Geometry check sheet. Reference: the model listing, model coordinates, mm. Round coordinates to 2 decimals unless told otherwise and drop trailing zeros. Write each loop counter-clockwise with the first axis right and the second up, starting at its lowest first coordinate (ties: lowest second). Pieces come first, ordered by that corner, then holes. Notation, with made-up numbers: (-31.5, -4.75) -> (11.5, -4.75) arc R27 cw to (11.5, 15.25) -> close; hole circle Ø6 at (-10, -8.75). An arc over 180 degrees is marked (long way). One line per question, with ' | ' between items.
Autodesk Inventor part; units mm, degrees
ref_plane "YZ Plane" through (0, 0, 0) normal (1, 0, 0) x (0, 1, 0)
ref_plane "XZ Plane" through (0, 0, 0) normal (0, 1, 0) x (-1, 0, 0)
ref_plane "XY Plane" through (0, 0, 0) normal (0, 0, 1) x (1, 0, 0)
sketch "Sketch1" plane through (0, 0, 0) normal (0, 0, 1) x (1, 0, 0)
  arc A0 (235.6827, -57.867) -> (240.6827, -52.867) centre (235.6827, -52.867) ccw
  line L0 (240.6827, -52.867) -> (240.6827, 24.133)
  arc A1 (240.6827, 24.133) -> (235.6827, 29.133) centre (235.6827, 24.133) ccw
  line L1 (235.6827, 29.133) -> (-24.3173, 29.133)
  arc A2 (-24.3173, 29.133) -> (-29.3173, 24.133) centre (-24.3173, 24.133) ccw
  line L2 (-29.3173, 24.133) -> (-29.3173, -52.867)
  arc A3 (-29.3173, -52.867) -> (-24.3173, -57.867) centre (-24.3173, -52.867) ccw
  line L3 (-24.3173, -57.867) -> (235.6827, -57.867)
  circle A4 centre (235.6827, 23.633) radius 1.7
  circle A5 centre (235.6827, -5.867) radius 1.7
  circle A6 centre (-24.3173, -5.867) radius 1.7
  circle A7 centre (-24.3173, 23.633) radius 1.7
  circle A8 centre (208.6827, 8.133) radius 2.75
  circle A9 centre (228.1827, -46.867) radius 3.3
  circle A10 centre (189.1827, -46.867) radius 3.3
  circle A11 centre (22.1827, -46.867) radius 3.3
  circle A12 centre (-16.8173, -46.867) radius 3.3
  circle A13 centre (235.6827, -5.867) radius 1.7
  circle A14 centre (235.6827, 23.633) radius 1.7
  circle A15 centre (-24.3173, 23.633) radius 1.7
  circle A16 centre (-24.3173, -5.867) radius 1.7
  arc A17 (235.6827, -57.867) -> (240.6827, -52.867) centre (235.6827, -52.867) ccw
  line L4 (240.6827, -52.867) -> (240.6827, 24.133)
  arc A18 (240.6827, 24.133) -> (235.6827, 29.133) centre (235.6827, 24.133) ccw
  line L5 (235.6827, 29.133) -> (172.1827, 29.133)
  arc A19 (-24.3173, 29.133) -> (-29.3173, 24.133) centre (-24.3173, 24.133) ccw
  line L6 (-29.3173, 24.133) -> (-29.3173, -52.867)
  arc A20 (-29.3173, -52.867) -> (-24.3173, -57.867) centre (-24.3173, -52.867) ccw
  line L7 (-24.3173, -57.867) -> (235.6827, -57.867)
  circle A21 centre (208.6827, 8.133) radius 2.75
  line L8 (221.1827, -40.867) -> (221.1827, -52.867)
  line L9 (221.1827, -52.867) -> (196.1827, -52.867)
  line L10 (196.1827, -52.867) -> (196.1827, -40.867)
  line L11 (196.1827, -40.867) -> (221.1827, -40.867)
  line L12 (-11.8173, -52.867) -> (-11.8173, -40.867)
  line L13 (-11.8173, -40.867) -> (15.1827, -40.867)
  line L14 (15.1827, -40.867) -> (15.1827, -52.867)
  line L15 (15.1827, -52.867) -> (-11.8173, -52.867)
  circle A22 centre (27.6827, -5.867) radius 1.7
  circle A23 centre (27.6827, 23.633) radius 1.7
  line L16 (172.1827, 29.133) -> (172.1827, -4.0741)
  line L17 (172.1827, -4.0741) -> (168.3898, -7.867)
  line L18 (168.3898, -7.867) -> (132.9756, -7.867)
  line L19 (132.9756, -7.867) -> (129.1827, -4.0741)
  line L20 (129.1827, -4.0741) -> (129.1827, 29.133)
  line L21 (129.1827, 29.133) -> (-24.3173, 29.133)
  circle A24 centre (181.6827, -5.867) radius 1.7
  circle A25 centre (181.6827, 23.633) radius 1.7
  circle A26 centre (1.6827, 8.133) radius 2.75
extrude "Extrusion1" add sketch "Sketch1" along normal blind 4 contours L3 A3 L2 A2 L1 L20 L19 L18 L17 L16 A1 L0 A0 | L16 L17 L18 L19 L20 L1 | A4 | A5 | A6 | A7 | A8 | A9 | A10 | A11 | A12 | A22 | A23 | A24 | A25 | A26
hole "Hole1" at (-24.3173, -5.867, 0) at (-24.3173, 23.633, 0) at (235.6827, 23.633, 0) at (235.6827, -5.867, 0) at (27.6827, 23.633, 0) at (27.6827, -5.867, 0) direction (0, 0, 1) diameter 3.4 end through all
hole "Hole2" at (208.6827, 8.133, 0) direction (0, 0, 1) diameter 5.5 end through all
hole "Hole3" at (-16.8173, -46.867, 0) at (22.1827, -46.867, 0) at (189.1827, -46.867, 0) at (228.1827, -46.867, 0) direction (0, 0, 1) diameter 3.4 end through all countersink diameter 6.6 countersink angle 90
sketch "Sketch2" plane through (0, 0, 4) normal (0, 0, 1) x (1, 0, 0)
  circle A0 centre (166.1827, -1.867) radius 1.7
  circle A1 centre (166.1827, 29.133) radius 1.7
  circle A2 centre (135.1827, 29.133) radius 1.7
  circle A3 centre (135.1827, -1.867) radius 1.7
  circle A4 centre (150.6827, 13.633) radius 11
  line L0 (168.1827, 34.633) -> (171.6827, 31.133)
  line L1 (168.1827, 34.633) -> (133.1827, 34.633)
  line L2 (129.6827, 31.133) -> (133.1827, 34.633)
  line L3 (129.6827, 31.133) -> (129.6827, -3.867)
  line L4 (133.1827, -7.367) -> (129.6827, -3.867)
  line L5 (133.1827, -7.367) -> (168.1827, -7.367)
  line L6 (171.6827, -3.867) -> (168.1827, -7.367)
  line L7 (171.6827, -3.867) -> (171.6827, 31.133)
  circle A5 centre (150.6827, 13.633) radius 11.5
  line L8 (150.6827, -7.367) -> (150.6827, -57.867)
  line L9 (-24.3173, -57.867) -> (235.6827, -57.867)
  line L10 (150.6827, -32.617) -> (163.331, -32.617) construction
  circle A6 centre (181.6827, 23.633) radius 1.7
  circle A7 centre (181.6827, -5.867) radius 1.7
  point P0 (0, 0)
  point P1 (150.6827, -17.367)
  point P2 (150.6827, -47.867)
  dimension "d23" = 0.5
  dimension "d35" = 10
extrude "Extrusion2" cut sketch "Sketch2" against normal through all contours A4 | A5
sketch "Sketch3" plane through (0, 0, 4) normal (0, 0, 1) x (1, 0, 0)
  circle A0 centre (166.1827, -1.867) radius 1.7
  circle A1 centre (166.1827, 29.133) radius 1.7
  circle A2 centre (135.1827, 29.133) radius 1.7
  circle A3 centre (135.1827, -1.867) radius 1.7
  circle A4 centre (150.6827, 13.633) radius 11
  line L0 (168.1827, 34.633) -> (171.6827, 31.133)
  line L1 (168.1827, 34.633) -> (133.1827, 34.633)
  line L2 (129.6827, 31.133) -> (133.1827, 34.633)
  line L3 (129.6827, 31.133) -> (129.6827, -3.867)
  line L4 (133.1827, -7.367) -> (129.6827, -3.867)
  line L5 (133.1827, -7.367) -> (168.1827, -7.367)
  line L6 (171.6827, -3.867) -> (168.1827, -7.367)
  line L7 (171.6827, -3.867) -> (171.6827, 31.133)
  line L8 (235.6827, 29.133) -> (-24.3173, 29.133)
  point P0 (0, 0)
  point P1 (129.6827, 29.133)
  point P2 (171.6827, 29.133)
extrude "Extrusion3" add sketch "Sketch3" against normal blind 4 contours L8 A1 | A1 L8 A2 L3 L2 L1 L0 L7 | L8 A2 picked at (166.251, 30.4471) picked at (135.251, 30.4471)
hole "Hole4" at (135.1827, -1.867, 4) at (135.1827, 29.133, 4) at (166.1827, 29.133, 4) at (166.1827, -1.867, 4) direction (0, 0, -1) diameter 3.4 end through all countersink diameter 6.6 countersink angle 90
sketch "Sketch4" plane through (0, 0, 0) normal (0, 0, -1) x (-1, 0, 0)
  point P0 (0, 0)
  point P1 (-150.6827, -17.367)
  point P2 (-150.6827, -47.867)
hole "Hole5" at (150.6827, -17.367, 0) at (150.6827, -47.867, 0) direction (0, 0, 1) diameter 4.3 end through all countersink diameter 8.6 countersink angle 90
hole "Hole6" at (181.6827, 23.633, 4) at (181.6827, -5.867, 4) direction (0, 0, -1) diameter 3.4 end through all countersink diameter 6.6 countersink angle 90
sketch "Sketch5" plane through (0, 0, 0) normal (0, 0, -1) x (-1, 0, 0)
  circle A0 centre (-17.1827, -7.367) radius 1.7
  circle A1 centre (-17.1827, 23.633) radius 1.7
  circle A2 centre (13.8173, 23.633) radius 1.7
  circle A3 centre (13.8173, -7.367) radius 1.7
  circle A4 centre (-1.6827, 8.133) radius 11
  line L0 (-19.1827, 29.133) -> (-22.6827, 25.633)
  line L1 (-19.1827, 29.133) -> (15.8173, 29.133)
  line L2 (19.3173, 25.633) -> (15.8173, 29.133)
  line L3 (19.3173, 25.633) -> (19.3173, -9.367)
  line L4 (15.8173, -12.867) -> (19.3173, -9.367)
  line L5 (15.8173, -12.867) -> (-19.1827, -12.867)
  line L6 (-22.6827, -9.367) -> (-19.1827, -12.867)
  line L7 (-22.6827, -9.367) -> (-22.6827, 25.633)
  point P0 (0, 0)
extrude "Extrusion4" cut sketch "Sketch5" against normal through all contours A4
hole "Hole7" at (17.1827, -7.367, 0) at (17.1827, 23.633, 0) at (-13.8173, 23.633, 0) at (-13.8173, -7.367, 0) direction (0, 0, 1) diameter 3.4 depth 8 countersink diameter 6.6 countersink angle 90
properties part number "plate_2"
(1) Sectioned sample at A-A on x = 202. Record the cut outline in (y, z), then the cut area to 3 significant figures.
Resolved:
outline: (-57.87, 0) -> (-52.87, 0) -> (-52.87, 4) -> (-57.87, 4) -> close; (-40.87, 0) -> (29.13, 0) -> (29.13, 4) -> (-40.87, 4) -> close | area: 300 mm2
(2) Sectioned sample at B-B on x = 62.5. Record the cut outline in (y, z).
Resolved:
outline: (-57.87, 0) -> (29.13, 0) -> (29.13, 4) -> (-57.87, 4) -> close
(3) Sectioned sample at C-C on z = 3.15. Count the separate pieces of the cut face and the enclosed holes in it, then the cut area to 3 significant figures.
Resolved:
separate pieces: 1 | enclosed holes: 27 | area: 22,000 mm2
(4) Material ranges on line 1 (X direction, y = -52, z = 1.55); line 2 (X direction, y = 31.5, z = 3.6); line 3 (Y direction, x = -11, z = 0.55), recorded low to high.
Resolved:
line 1: x = -29.32 to -11.82, 15.18 to 196.18, 221.18 to 240.68 | line 2: x = 130.05 to 133.51, 136.86 to 164.51, 167.86 to 171.32 | line 3: y = -57.87 to -52.87, -40.87 to 29.13
(5) Go/stop test with a flat-tipped pin: pin 1 (5.5 mm diameter, centred on x = -16.82, y = -46.87, fed in from -Z). Record where the tip stops, or that it passes through.
Resolved:
pin 1: stops at z = 0.55
(6) Draft check along X on faces 1 (the cylindrical face through (152.782, -17.833, 3.088)), 2 (the cylindrical face through (239.26, -56.36, 1.97)), 3 (the flat face through (104, -11, 4)). Enter one of: +X half, -X half, draft (parallel to the pull), parting line (faces both ways), or undercut.
Resolved:
face 1: undercut | face 2: +X half | face 3: draft
